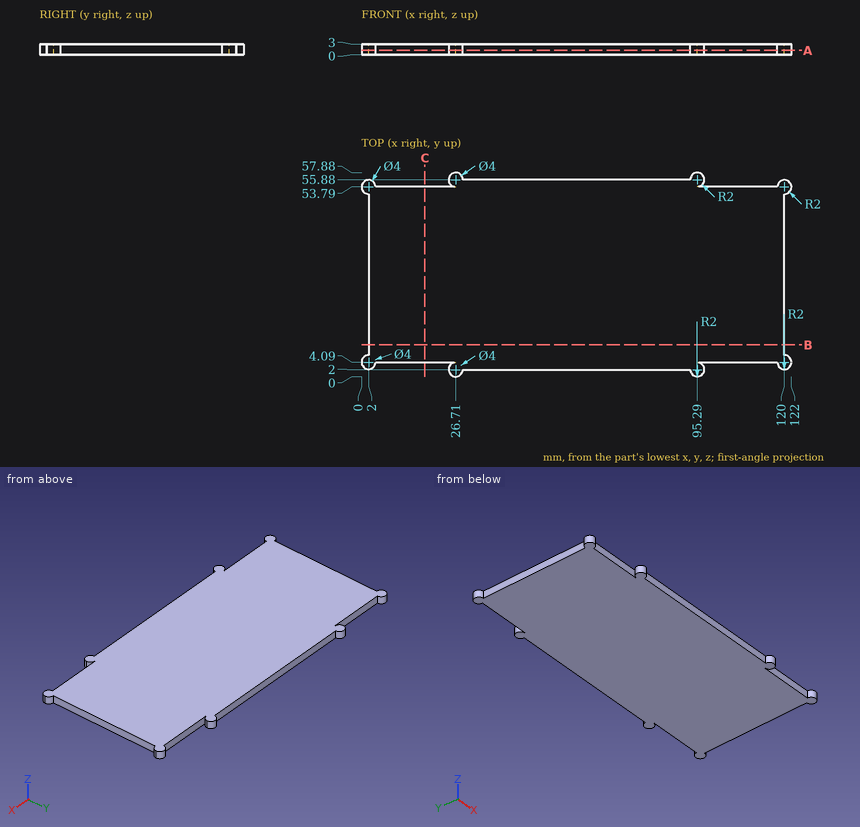
The figure shows three views and two pictorial views of one solid part (mm, origin at its lowest corner). Answer the questions. Coordinates: 2 decimals unless noted, no trailing zeros. Loops run counter-clockwise (first coordinate to the right, second up) from the corner with the lowest first, then second, coordinate; pieces in that order, holes last. Notation, with made-up numbers: M -22,69.25 L 30,69.25 A22 cw 30,105.25 Z; hole C 35.25,18.5 d3. An arc over 180 degrees is marked long. Use CSV: the item, a comma, the result in double quotes. Start each with the question number.
(1) Find section C-C, the plane x = 18. Give the vertices of the cut face in (y, z).
(2) Find section B-B, the plane y = 9. Give the vertices of the cut face in (x, z).
(3) Consider line 1 (X direction, y = 3, z = 2.1); line 2 (X direction, y = 43, z = 0.65); line 3 (Y direction, x = 19, z = 2.7). Determine where each line is inside the solid, lowest interval first.
(4) Given pin 1 Ø1 at (x, z) = (108, 1) entering from +Y; pin 2 Ø1.5 at (x, z) = (15.5, 1.5) entering from -Y; pin 3 Ø1 at (x, z) = (86, 1.5) entering from -Y; pin 4 Ø2 at (x, y) = (33, 16) entering from -Z, each flat-ended and moving along its own axis, determine where each tip first touches the part or whether it passes through.
(5) Find section A-A, the plane z = 1.2. Give the vertices of the cut face in (x, y), then the cut area to 3 significant figures.
Recorded:
1,outline,"M 4.09,0 L 53.79,0 L 53.79,3 L 4.09,3 Z"
2,outline,"M 2,0 L 120,0 L 120,3 L 2,3 Z"
3,line 1,"x = 0.32 to 3.68, 24.98 to 97.02, 118.32 to 121.68"
3,line 2,"x = 2 to 120"
3,line 3,"y = 4.09 to 53.79"
4,pin 1,"stops at y = 53.79"
4,pin 2,"stops at y = 4.09"
4,pin 3,"stops at y = 2"
4,pin 4,"stops at z = 0"
5,outline,"M 2,6.09 A2 ccw long 4,4.09 L 26.71,4.09 L 26.71,4 A2 ccw long 28.71,2 L 93.29,2 A2 ccw long 95.29,4 L 95.29,4.09 L 118,4.09 A2 ccw long 120,6.09 L 120,51.79 A2 ccw long 118,53.79 L 95.29,53.79 L 95.29,53.88 A2 ccw long 93.29,55.88 L 28.71,55.88 A2 ccw long 26.71,53.88 L 26.71,53.79 L 4,53.79 A2 ccw long 2,51.79 Z"
5,area,"6,230 mm^2"
